Autodesk Inventor part; units mm, degrees
ref_plane "YZ Plane" through (0, 0, 0) normal (1, 0, 0) x (0, 1, 0)
ref_plane "XZ Plane" through (0, 0, 0) normal (0, 1, 0) x (-1, 0, 0)
ref_plane "XY Plane" through (0, 0, 0) normal (0, 0, 1) x (1, 0, 0)
sketch "Sketch1" plane through (0, 0, 0) normal (0, 0, 1) x (1, 0, 0)
  line L0 (-32.6, -32.6) -> (32.6, -32.6)
  line L1 (32.6, -32.6) -> (32.6, 32.6)
  line L2 (32.6, 32.6) -> (-32.6, 32.6)
  line L3 (-32.6, 32.6) -> (-32.6, -32.6)
  line L4 (-32.6, -32.6) -> (32.6, 32.6) construction
  line L5 (32.6, -32.6) -> (-32.6, 32.6) construction
  point P0 (0, 0)
  dimension "d0" = 65.2
  dimension "d1" = 65.2
extrude "Extrusion1" add sketch "Sketch1" along normal blind 1
sketch "Sketch2" plane through (0, 0, 1) normal (0, 0, 1) x (1, 0, 0)
  circle A0 centre (-29.6, 14.557) radius 1.575
  circle A1 centre (29.525, 18.595) radius 1.575
  circle A2 centre (29.583, -21.6) radius 1.575
  line L0 (-32.6, 32.6) -> (-32.6, -32.6)
  line L1 (32.6, 32.6) -> (-32.6, 32.6)
  line L2 (32.6, -32.6) -> (32.6, 32.6)
  line L3 (-32.6, -32.6) -> (32.6, -32.6)
  point P0 (0, 0)
  dimension "d4" = 3
  dimension "d5" = 18.043
  dimension "d6" = 3.075
  dimension "d7" = 14.005
  dimension "d8" = 11
  dimension "d9" = 3.017
  dimension "d10" = 3.15
  dimension "d11" = 3.15
  dimension "d12" = 3.15
extrude "Extrusion2" cut sketch "Sketch2" against normal blind 1 contours A0 | A1 | A2
properties part number "PCB"
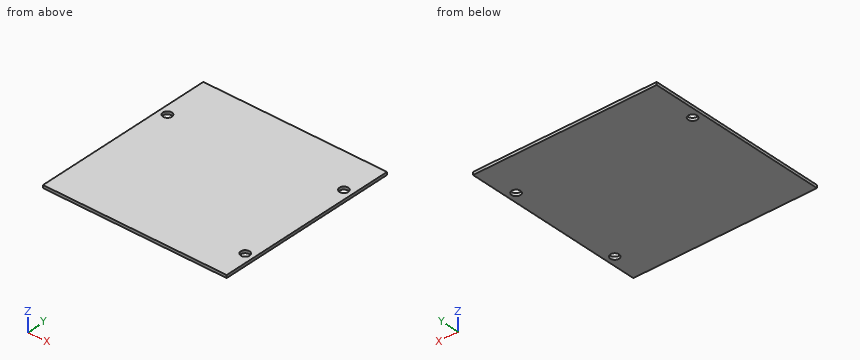
Part model, mm, in its own coordinate system. Round coordinates to 2 decimals unless told otherwise and drop trailing zeros. Write each loop counter-clockwise with the first axis right and the second up, starting at its lowest first coordinate (ties: lowest second). Pieces come first, ordered by that corner, then holes. Notation, with made-up numbers: M 73.5,17 L 88.5,17 A11 cw 88.5,31 Z; hole C 46,87 d11. An arc over 180 degrees is marked long. Return JSON: item names as keys, results as strings. Group by question number.
(1) Saw through at A-A on y = -21.6. Write the cut outline in (x, z), then the cut area to 4 significant figures.
(2) Saw through at B-B on x = -29.6. Write the cut outline in (y, z).
(3) Drill centre lines: probe 1 along Y at (x, z) = (-29.6, 0.5); probe 2 along X at (y, z) = (17.5, 0.55); probe 3 along X at (y, z) = (16, 0.3). Where is each one in solid material? Low to high.
Returned:
{
 "1": {"outline": "M -32.6,0 L 28.01,0 L 28.01,1 L -32.6,1 Z; M 31.16,0 L 32.6,0 L 32.6,1 L 31.16,1 Z", "area": "62.05 mm²"},
 "2": {"outline": "M -32.6,0 L 12.98,0 L 12.98,1 L -32.6,1 Z; M 16.13,0 L 32.6,0 L 32.6,1 L 16.13,1 Z"},
 "3": {"probe 1": "-32.6 to 12.98, 16.13 to 32.6", "probe 2": "-32.6 to 28.39, 30.66 to 32.6", "probe 3": "-32.6 to -30.23, -28.97 to 32.6"}
}
